Source: CAD feature listing. Evaluate the final solid. Frame: model axes, mm. Round coordinates to 2 decimals unless told otherwise and drop trailing zeros. Loops run counter-clockwise (first coordinate to the right, second up) from the corner with the lowest first, then second, coordinate; pieces in that order, holes last. Notation, with made-up numbers: M 57.25,61.25 L 71.25,61.25 A6 cw 71.25,68.25 Z; hole C 69.25,18 d11. An arc over 180 degrees is marked long. Answer as a JSON object with one key per item and string values.
Autodesk Inventor part; units mm, degrees
ref_plane "Work Plane1" through (0, 0, 0) normal (1, 0, 0) x (0, 0, 1)
ref_plane "XZ Plane" through (0, 0, 0) normal (0, 1, 0) x (-1, 0, 0)
ref_plane "XY Plane" through (0, 0, 0) normal (0, 0, 1) x (1, 0, 0)
sketch "Sketch1" plane through (0, 0, 0) normal (0, 0, 1) x (1, 0, 0)
  circle A0 centre (0, 0) radius 21.0312
  circle A1 centre (0, 0) radius 17.4625
  dimension "d0" = 42.0624
  dimension "d1" = 34.925
extrude "Extrusion1" add sketch "Sketch1" along normal mid plane 965.2
ref_plane "Work Plane1" through (0, 0, 0) normal (1, 0, 0) x (0, 0, 1)
sketch "Sketch2" plane through (0, 0, 0) normal (1, 0, 0) x (0, 0, 1)
  line L0 (-482.6, -21.0312) -> (482.6, -21.0312)
  line L1 (-482.6, 21.0312) -> (482.6, 21.0312)
  line L2 (482.6, 17.4625) -> (482.6, -17.4625)
  line L3 (482.6, 21.0312) -> (482.6, -21.0312)
  line L4 (-482.6, -17.4625) -> (-482.6, 17.4625)
  line L5 (-482.6, -21.0312) -> (-482.6, 21.0312)
  line L6 (-675.64, 0) -> (675.64, 0)
  arc A0 (474.6625, -3.175) -> (474.6625, 3.175) centre (474.6625, 0) ccw
  arc A1 (436.5625, -3.175) -> (436.5625, 3.175) centre (436.5625, 0) ccw
  arc A2 (461.9625, 3.175) -> (461.9625, -3.175) centre (461.9625, 0) ccw
  arc A3 (423.8625, 3.175) -> (423.8625, -3.175) centre (423.8625, 0) ccw
  line L7 (423.8625, 3.175) -> (436.5625, 3.175)
  line L8 (423.8625, -3.175) -> (436.5625, -3.175)
  line L9 (461.9625, -3.175) -> (474.6625, -3.175)
  line L10 (461.9625, 3.175) -> (474.6625, 3.175)
  dimension "d5" = 7.9375
  dimension "d6" = 38.1
  dimension "d7" = 6.35
  dimension "d18" = 12.7
  dimension "d19" = 12.7
extrude "Extrusion2" cut sketch "Sketch2" against normal blind 965.2 contours A3 L7 A1 L6 | L6 A1 L8 A3 | A0 L9 A2 L6 | L6 A2 L10 A0
sketch "Sketch3" plane through (0, 0, 0) normal (1, 0, 0) x (0, 0, 1)
  line L0 (-298.45, -3.175) -> (-450.85, -3.175)
  line L1 (-454.025, 0) -> (-454.025, 6.35)
  line L2 (-450.85, 9.525) -> (-450.85, 9.525)
  line L3 (-447.675, 6.35) -> (-447.675, 3.175)
  line L4 (-447.675, 3.175) -> (-298.45, 3.175)
  arc A0 (-298.45, -3.175) -> (-298.45, 3.175) centre (-298.45, 0) ccw
  arc A1 (-450.85, 9.525) -> (-454.025, 6.35) centre (-450.85, 6.35) ccw
  arc A2 (-447.675, 6.35) -> (-450.85, 9.525) centre (-450.85, 6.35) ccw
  arc A3 (-454.025, 0) -> (-450.85, -3.175) centre (-450.85, 0) ccw
  line L5 (-482.6, -21.0312) -> (-482.6, 21.0312)
  line L6 (-675.64, 0) -> (675.64, 0)
  dimension "d10" = 6.35
  dimension "d11" = 6.35
  dimension "d12" = 3.175
  dimension "d13" = 6.35
  dimension "d14" = 152.4
  dimension "d15" = 31.75
extrude "Extrusion3" cut sketch "Sketch3" along normal blind 965.2
properties part number "FE-00028"
Item 1: Pull-direction query (Y, two-part tool) for faces 1 (the cylindrical face through (16.656, 5.245, 6.756)), 2 (the flat face through (-8, 16, -482.6)), 3 (the cylindrical face through (20.06, -6.32, -6.76)); classes: pulls with the +Y half, pulls with the -Y half, needs draft (parallel to the pull), parting line crosses it, or undercut.
Answer sheet:
{"face 1": "undercut", "face 2": "needs draft", "face 3": "parting line crosses it"}
Item 2: Section B-B on z = 23. Return the cut outline in (x, y) (1 decimal), then the cut area to 3 significant figures.
Answer sheet:
{"outline": "C 0,0 d42.1; hole C 0,0 d34.9", "area": "432 mm²"}
Item 3: Contact query for flat-ended pins moving along their axis: pin 1 Ø4 at (x, z) = (-18, 470) entering from -Y; pin 2 Ø4 at (x, z) = (-19, 429) entering from -Y; pin 3 Ø1.1 at (x, z) = (18, -396) entering from +Y. Output: stop coordinate, or through.
Answer sheet:
{"pin 1": "stops at y = -13.65", "pin 2": "stops at y = -12.38", "pin 3": "stops at y = 11.74"}
Item 4: Section A-A on x = 4. Return the cut outline in (y, z), then the cut area to 3 significant figures.
Answer sheet:
{"outline": "M -20.65,-482.6 L -17,-482.6 L -17,482.6 L -20.65,482.6 Z; M 17,-482.6 L 20.65,-482.6 L 20.65,482.6 L 17,482.6 Z", "area": "7,040 mm²"}
Item 5: Line query: probe 1 along X at (y, z) = (0, -228.5); probe 2 along Y at (x, z) = (-1, -164.5). Output: solid intervals per line, ascending. Write a range as from..to.
Answer sheet:
{"probe 1": "x = -21.03..-17.46, 17.46..21.03", "probe 2": "y = -21.01..-17.43, 17.43..21.01"}
